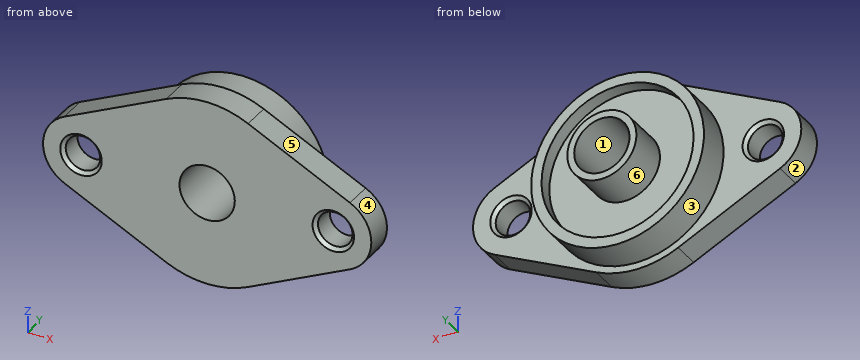
```python
from build123d import *

# Parameters (mm, degrees)
CROQUIS1_R              = 4
CROQUIS1_R_2            = 2.5
SALIENTE_EXTRUIR1_DEPTH = 4
CROQUIS2_R              = 5
CROQUIS2_R_2            = 4
SALIENTE_EXTRUIR2_DEPTH = 9
CROQUIS3_R              = 12.5
CROQUIS3_R_2            = 11
SALIENTE_EXTRUIR3_DEPTH = 5
CROQUIS5_R              = 11
CROQUIS5_R_2            = 5
SALIENTE_EXTRUIR4_DEPTH = 3
CHAFL_N1_SIZE           = 0.5


with BuildPart() as part:
    # Croquis1 → Saliente-Extruir1 (new body)
    with BuildSketch(Plane(origin=(0, 0, 0), x_dir=(1, 0, 0), z_dir=(0, 1, 0))):
        with BuildLine():
            Line((-5.917808219, 12.133818273), (-20.660958904, 4.943407445))
            ThreePointArc((-20.660958904, 4.943407445), (-23.75, 0), (-20.660958904, -4.943407445))
            Line((-20.660958904, -4.943407445), (-5.917808219, -12.133818273))
            ThreePointArc((-5.917808219, -12.133818273), (0, -13.5), (5.917808219, -12.133818273))
            Line((5.917808219, -12.133818273), (20.660958904, -4.943407445))
            ThreePointArc((20.660958904, -4.943407445), (23.75, 0), (20.660958904, 4.943407445))
            Line((20.660958904, 4.943407445), (5.917808219, 12.133818273))
            ThreePointArc((5.917808219, 12.133818273), (0, 13.5), (-5.917808219, 12.133818273))
        make_face()
        with Locations(Location((0, 0, 0), (0, 0, 270))):
            Circle(CROQUIS1_R, mode=Mode.SUBTRACT)
        with Locations(Location((-18.25, 0, 0), (0, 0, 270))):
            Circle(CROQUIS1_R_2, mode=Mode.SUBTRACT)
        with Locations(Location((18.25, 0, 0), (0, 0, 270))):
            Circle(CROQUIS1_R_2, mode=Mode.SUBTRACT)
    extrude(amount=SALIENTE_EXTRUIR1_DEPTH)

    # Croquis2 → Saliente-Extruir2 (add)
    with BuildSketch(Plane(origin=(0, 4, 0), x_dir=(1, 0, 0), z_dir=(0, 1, 0))):
        with Locations(Location((0, 0, 0), (0, 0, 270))):
            Circle(CROQUIS2_R)
        with Locations(Location((0, 0, 0), (0, 0, 270))):
            Circle(CROQUIS2_R_2, mode=Mode.SUBTRACT)
    extrude(amount=SALIENTE_EXTRUIR2_DEPTH)

    # Croquis3 → Saliente-Extruir3 (add)
    with BuildSketch(Plane(origin=(0, 4, 0), x_dir=(1, 0, 0), z_dir=(0, 1, 0))):
        with Locations(Location((0, 0, 0), (0, 0, 270))):
            Circle(CROQUIS3_R)
        with Locations(Location((0, 0, 0), (0, 0, 270))):
            Circle(CROQUIS3_R_2, mode=Mode.SUBTRACT)
    extrude(amount=SALIENTE_EXTRUIR3_DEPTH)

    # Croquis5 → Saliente-Extruir4 (add)
    with BuildSketch(Plane(origin=(0, 4, 0), x_dir=(1, 0, 0), z_dir=(0, 1, 0))):
        with Locations(Location((0, 0, 0), (0, 0, 270))):
            Circle(CROQUIS5_R)
        with Locations(Location((0, 0, 0), (0, 0, 270))):
            Circle(CROQUIS5_R_2, mode=Mode.SUBTRACT)
    extrude(amount=SALIENTE_EXTRUIR4_DEPTH)

    # Chaflán1
    chafl_n1_edges = [part.edges().sort_by_distance(p)[0] for p in [
        (-18.25, 0, -2.5),
        (-18.25, 4, -2.5),
        (18.25, 0, -2.5),
        (18.25, 4, -2.5),
    ]]
    chamfer(chafl_n1_edges, length=CHAFL_N1_SIZE)


solid = part.part
```
Part model, mm, in its own coordinate system. Face numbers are marked on the shaded views. A direction names the side the tool comes from. Coordinates: 2 decimals unless noted, no trailing zeros. Write each loop counter-clockwise with the first axis right and the second up, starting at its lowest first coordinate (ties: lowest second). Pieces come first, ordered by that corner, then holes.
Item 1: Which spindle directions (+Z, -Z, +X, -X, +Y, -Y) get a long thin tool onto all of the face, cutting with end or side? Do the marked faces 5 and 6. Say none if no direction does.
Item 2: Pin check, flat tips, straight feed: pin 1 (4.5 mm diameter, centred on x = 18.25, z = 0, fed in from -Y); pin 2 (3 mm diameter, centred on y = 7.5, z = 1.5, fed in from -X); pin 3 (5 mm diameter, centred on x = 14, z = -7, fed in from +Y); pin 4 (12 mm diameter, centred on x = -13, z = 6.5, fed in from +Y). Stop position of each tip, or through.
Item 3: Slice it at B-B (y = 8). Write the cut outline in (x, z).
Item 4: Slice it at A-A (x = 0). Write the cut outline in (y, z), and give its area (3 significant figures).
Item 5: Slice it at C-C (z = 0). Count the separate pieces of the cut face and the enclosed holes in it, and give its area (3 significant figures).
Item 6: Slice it at D-D (z = 7.25). Write the cut outline in (x, y).
Item 7: Probe line 1 (X direction, y = 3.5, z = 0); line 2 (X direction, y = 8.45, z = 0); line 3 (X direction, y = 6.75, z = 0). List the from-to ranges inside material, lowest first.
Item 8: Mould opens along X. For the marked faces 1, 2, 3 and 4 say: released by +X, released by -X, zero draft, split by the parting line, or undercut.
Results found:
1. face 5: +Z, +X, +Y, -Y
1. face 6: +Y
2. pin 1: passes through
2. pin 2: stops at x = -12.5
2. pin 3: stops at y = 4
2. pin 4: stops at y = 9
3. outline: circle Ø25 at (0, 0); circle Ø10 at (0, 0); hole circle Ø22 at (0, 0); hole circle Ø8 at (0, 0)
4. outline: (0, -13.5) - (4, -13.5) - (4, -12.5) - (9, -12.5) - (9, -11) - (7, -11) - (7, -5) - (13, -5) - (13, -4) - (0, -4) - close; (0, 4) - (13, 4) - (13, 5) - (7, 5) - (7, 11) - (9, 11) - (9, 12.5) - (4, 12.5) - (4, 13.5) - (0, 13.5) - close
4. area: 145 mm2
5. separate pieces: 4
5. enclosed holes: 0
5. area: 186 mm2
6. outline: (-15.93, 0) - (15.93, 0) - (15.93, 4) - (10.18, 4) - (10.18, 9) - (8.27, 9) - (8.27, 7) - (-8.27, 7) - (-8.27, 9) - (-10.18, 9) - (-10.18, 4) - (-15.93, 4) - close
7. line 1: x = -23.75 to -20.75, -15.75 to -4, 4 to 15.75, 20.75 to 23.75
7. line 2: x = -12.5 to -11, -5 to -4, 4 to 5, 11 to 12.5
7. line 3: x = -12.5 to -4, 4 to 12.5
8. face 1: undercut
8. face 2: released by -X
8. face 3: split by the parting line
8. face 4: released by +X
